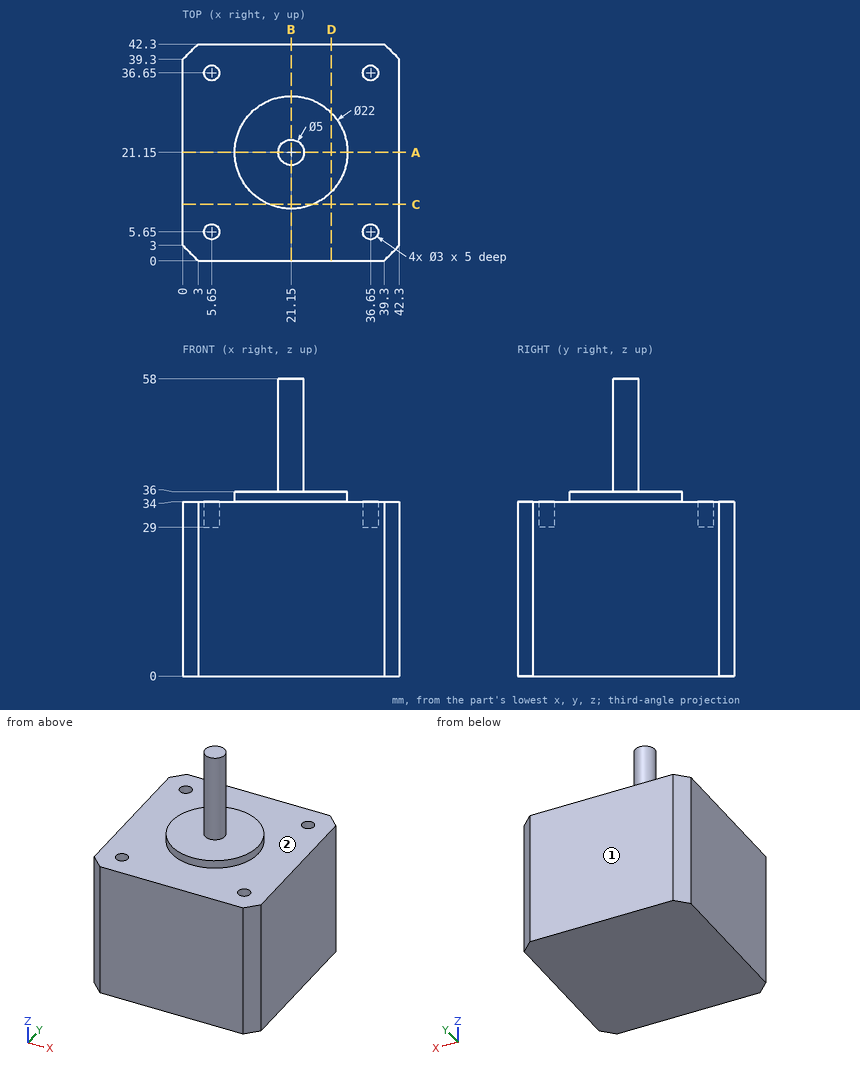
Design review of the part shown in the three views and the two pictorial views. Dimensions are in mm from the part's minimum x, y and z. A direction names the side the tool comes from. Round coordinates to 2 decimals unless told otherwise and drop trailing zeros. Write each loop counter-clockwise with the first axis right and the second up, starting at its lowest first coordinate (ties: lowest second). Pieces come first, ordered by that corner, then holes. Notation, with made-up numbers: (2, 63) - (61, 63) arc R16 cw to (61, 73) - close; hole circle Ø11 at (-8, 60.25). An arc over 180 degrees is marked (long way). Write item = value, one per line. Start each with the question number.
1. Consider section A-A on y = 21.15. State the section outline as (x, z) points.
2. For the marked faces 1 and 2, list the 3-axis set-ups (+Z, -Z, +X, -X, +Y, -Y) from which the entire face can be reached by the end or side of a thin tool; tool diameter is ignored.
3. Wall thickness on L1, parallel to Y at x = 5.65, z = 32.7; L2, parallel to Y at x = 36, z = 33; L3, parallel to Z at x = 5, y = 29.5: over which ranges is each line inside the solid? List them lowest first.
4. Consider section D-D on x = 29. State the section outline as (y, z) points.
5. Consider section C-C on y = 11. State the section outline as (x, z) points, plus the area to 3 significant figures.
6. For pin 1 Ø3.5 at (x, y) = (36.5, 5) entering from +Z; pin 2 Ø12 at (y, z) = (12, 35.5) entering from -X; pin 3 Ø1.5 at (x, y) = (5.5, 5.5) entering from +Z; pin 4 Ø10 at (x, y) = (11.5, 16) entering from +Z, all flat-tipped, find the tip position at first contact; note any pin that passes through.
Evaluation:
q1.outline = (0, 0) - (42.3, 0) - (42.3, 34) - (32.15, 34) - (32.15, 36) - (23.65, 36) - (23.65, 58) - (18.65, 58) - (18.65, 36) - (10.15, 36) - (10.15, 34) - (0, 34) - close
q2.face_1 = +Z, -Z, +X, -X, +Y
q2.face_2 = +Z
q3.L1 = 0 to 4.15, 7.15 to 35.15, 38.15 to 42.3
q3.L2 = 0 to 4.3, 7 to 35.3, 38 to 42.3
q3.L3 = 0 to 34
q4.outline = (0, 0) - (42.3, 0) - (42.3, 34) - (28.86, 34) - (28.86, 36) - (13.44, 36) - (13.44, 34) - (0, 34) - close
q5.outline = (0, 0) - (42.3, 0) - (42.3, 34) - (25.39, 34) - (25.39, 36) - (16.91, 36) - (16.91, 34) - (0, 34) - close
q5.area = 1,460 mm2
q6.pin_1 = 34
q6.pin_2 = 0
q6.pin_3 = 29
q6.pin_4 = 36
